Verification items for the finished model (mm, model axes). A direction names the side the tool comes from. Round coordinates to 2 decimals unless told otherwise and drop trailing zeros. Write each loop counter-clockwise with the first axis right and the second up, starting at its lowest first coordinate (ties: lowest second). Pieces come first, ordered by that corner, then holes. Notation, with made-up numbers: M -12.5,64 L 14.5,64 A6 cw 14.5,73 Z; hole C 14,82.5 d5. An arc over 180 degrees is marked long. Answer in a Markdown table with one row per item. Add a question column.
1. Set-up check for faces 1 (the cylindrical face through (-3.236, 0.031, 1.493)), 2 (the flat face through (-0.2, 2, 0)), 3 (the cylindrical face through (8, 0, 0)), 4 (the cylindrical face through (-3.236, 0.031, -1.507)), 5 (the cylindrical face through (11.764, 0.031, 1.493)): record each of +Z, -Z, +X, -X, +Y, -Y from which the full face is reachable in a straight line by a thin tool's end or side.
2. Go/stop test with flat-tipped pins: pin 1 Ø1.5 at (x, y) = (-13.5, 1) entering from +Z; pin 2 Ø2 at (x, y) = (15, 0) entering from +Z; pin 3 Ø1.5 at (y, z) = (-1, 0) entering from +X; pin 4 Ø2 at (x, y) = (6, -0.5) entering from -Z. Record where each tip stops, or that it passes through.
3. Sectioned sample at A-A on z = -0.1. Record the cut outline in (x, y).
4. Draft check along Z on faces 6 (the cylindrical face through (1, 0, 0)), 7 (the flat face through (-0.2, -2, 0)), 8 (the flat face through (-10, 0, -1)). Enter one of: pulls with the +Z half, pulls with the -Z half, needs draft (parallel to the pull), parting line crosses it, or undercut.
5. Sectioned sample at D-D on z = -1.65. Record the cut outline in (x, y).
6. Material ranges on probe 1 along X at (y, z) = (0, -0.35); probe 2 along Y at (x, z) = (15, 0.25); probe 3 along Z at (x, y) = (7, -0.45), recorded low to high.
7. Sectioned sample at C-C on y = 0. Count the separate pieces of the cut face and the enclosed holes in it, plus the area to 3 significant figures.
8. Sectioned sample at B-B on x = 5. Record the cut outline in (y, z).
Autodesk Inventor part; units mm, degrees
ref_plane "YZ Plane" through (0, 0, 0) normal (1, 0, 0) x (0, 1, 0)
ref_plane "XZ Plane" through (0, 0, 0) normal (0, 1, 0) x (-1, 0, 0)
ref_plane "XY Plane" through (0, 0, 0) normal (0, 0, 1) x (1, 0, 0)
sketch "Sketch1" plane through (0, 0, 0) normal (0, 0, 1) x (1, 0, 0)
  line L0 (0, 0) -> (15, 0)
  line L1 (0, 0) -> (-15, 0)
  line L2 (0, 0) -> (5, 0)
  circle A0 centre (-15, 0) radius 1.25
  circle A1 centre (15, 0) radius 1.25
  circle A2 centre (-15, 0) radius 2
  circle A3 centre (15, 0) radius 2
  line L3 (-15, 2) -> (15, 2)
  line L4 (-15, -2) -> (15, -2)
  circle A4 centre (5, 0) radius 1.25
  line L5 (-15, 2) -> (-4, 2)
  line L6 (-4, 2) -> (-4, -2)
  line L7 (-4, -2) -> (-15, -2)
  line L8 (-15, -2) -> (-15, 2)
  line L9 (15, 2) -> (12.5, 2)
  line L10 (12.5, -2) -> (15, -2)
  line L11 (15, -2) -> (15, 2)
  line L12 (15, 2) -> (14.5, 2)
  line L13 (15, -2) -> (14.5, -2)
  arc A5 (-4, -2) -> (-4, 2) centre (-6.2361, 0) ccw
  line L14 (5, 0) -> (1, 0)
  arc A6 (0, -2) -> (0, 2) centre (-1.5, 0) ccw
  line L15 (0, 2) -> (0, -2)
  line L16 (5, 2) -> (9, 2)
  line L17 (9, 2) -> (9, -2)
  line L18 (5, 0) -> (8, 0)
  arc A7 (9, 2) -> (9, -2) centre (10.5, 0) ccw
  line L19 (-15, 2) -> (-14.5, 2)
  line L20 (-15, -2) -> (-14.5, -2)
  arc A8 (-14.5, -2) -> (-14.5, 2) centre (-14.5, 0) ccw
  line L21 (9, 2) -> (11, 2)
  line L22 (9, -2) -> (11, -2)
  arc A9 (11, -2) -> (11, 2) centre (8.7639, 0) ccw
  point P0 (-4, 2)
  dimension "d1" = 15
  dimension "d2" = 15
  dimension "d3" = 5
  dimension "d4" = 2.5
  dimension "d6" = 2.5
  dimension "d7" = 4
  dimension "d8" = 4
  dimension "d9" = 2.5
  dimension "d10" = 11
  dimension "d16" = 4
  dimension "d17" = 3
  dimension "d18" = 4
  dimension "d21" = 4
  dimension "d23" = 3
  dimension "d24" = 0.5
  dimension "d25" = 0.5
  dimension "d26" = 2
  dimension "d35" = 2
  dimension "d36" = 2
  dimension "d37" = 3
  dimension "d38" = 4
extrude "Extrusion1" add sketch "Sketch1" along normal mid plane 2 contours A5 L6 L1 | L1 L6 A5 | L6 L4 A8 L1 | L1 A8 L3 L6 | A8 L4 A2 L1 | L1 A2 L3 A8 | A9 L0 A3 L4 | A2 L8 A0 L1 | L1 A0 L8 A2 | A2 L8 A0 | L3 A3 L0 A9 | A3 L11 A1 L0 | L0 A1 L11 A3 | L11 A1 A3
extrude "Extrusion2" add sketch "Sketch1" along normal mid plane 4 contours L15 A6 L0 | L15 L4 A5 L1 | L1 A5 L3 L15 | L0 A6 L15 | L17 L0 A9 L4 | A7 L0 L17 | L3 A9 L0 L17 | L17 L0 A7
extrude "Extrusion3" add sketch "Sketch1" along normal mid plane 4 contours A6 L3 A7 L0 A4 | L0 A4 A7 L4 A6
extrude "Extrusion4" cut sketch "Sketch1" along normal mid plane 2 contours A6 L3 A7 L0 A4 | L0 A4 A7 L4 A6
properties part number "link7" material "Aluminum 6061"
Geometry check:
| question | item | result |
|---|---|---|
| 1 | face 1 | +Z, -X |
| 1 | face 2 | +Z, -Z, +X, -X, +Y |
| 1 | face 3 | none |
| 1 | face 4 | -Z, -X |
| 1 | face 5 | +Z, +X |
| 2 | pin 1 | stops at z = 1 |
| 2 | pin 2 | passes through |
| 2 | pin 3 | stops at x = 16.98 |
| 2 | pin 4 | stops at z = -2 |
| 3 | outline | M -15,-2 L 0,-2 A2.5 ccw 0,2 L -15,2 A2 ccw Z; M 9,-2 L 15,-2 A2 ccw 15,2 L 9,2 A2.5 ccw Z; hole C -15,0 d2.5; hole C 15,0 d2.5 |
| 4 | face 6 | undercut |
| 4 | face 7 | needs draft |
| 4 | face 8 | pulls with the -Z half |
| 5 | outline | M -4,-2 L 11,-2 A3 ccw 11,2 L -4,2 A3 cw Z; hole C 5,0 d2.5 |
| 6 | probe 1 | x = -17 to -16.25, -13.75 to 1, 8 to 13.75, 16.25 to 17 |
| 6 | probe 2 | y = -2 to -1.25, 1.25 to 2 |
| 6 | probe 3 | z = -2 to -1, 1 to 2 |
| 7 | separate pieces | 4 |
| 7 | enclosed holes | 0 |
| 7 | area | 69.0 mm2 |
| 8 | outline | M -2,-2 L -1.25,-2 L -1.25,-1 L -2,-1 Z; M -2,1 L -1.25,1 L -1.25,2 L -2,2 Z; M 1.25,-2 L 2,-2 L 2,-1 L 1.25,-1 Z; M 1.25,1 L 2,1 L 2,2 L 1.25,2 Z |
